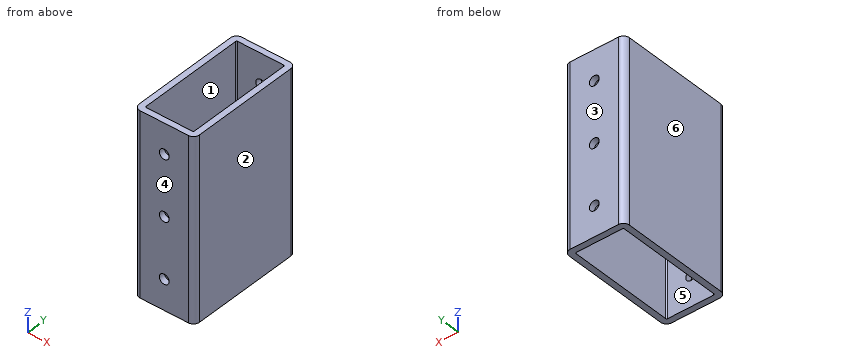
```python
from build123d import *

# Parameters (mm, degrees)
SKETCH1_W                 = 76.2
SKETCH1_H                 = 50.8
BOSS_EXTRUDE1_DEPTH       = 25.4
SKETCH2_W                 = 20.32
SKETCH2_H                 = 45.72
CUT_EXTRUDE1_DEPTH        = 77.2
F_6_CLEARANCE_HOLE1_D     = 4.1402
F_6_CLEARANCE_HOLE1_DEPTH = 50.8
F_6_CLEARANCE_HOLE2_D     = 4.1402
F_6_CLEARANCE_HOLE2_DEPTH = 50.8
FILLET1_R                 = 0.5
FILLET2_R                 = 2.54


with BuildPart() as part:
    # Sketch1 → Boss-Extrude1 (new body)
    with BuildSketch(Plane(origin=(12.7, 0, 0), x_dir=(0, 0, -1), z_dir=(1, 0, 0))):
        Rectangle(SKETCH1_W, SKETCH1_H)
    extrude(amount=-BOSS_EXTRUDE1_DEPTH)

    # Sketch2 → Cut-Extrude1 (cut, through all)
    with BuildSketch(Plane(origin=(0, 0, -38.1), x_dir=(-1, 0, 0), z_dir=(0, 0, -1))):
        Rectangle(SKETCH2_W, SKETCH2_H)
    extrude(amount=-CUT_EXTRUDE1_DEPTH, mode=Mode.SUBTRACT)

    # #6 Clearance Hole1
    with Locations(Plane(origin=(0, -25.4, 0), x_dir=(-1, 0, 0), z_dir=(0, -1, 0))):
        with Locations((0, 711.2), (0, 736.6), (0, 685.8), (0, 660.4), (0, 635), (0, 609.6), (0, 584.2), (0, 558.8), (0, 533.4), (0, 508), (0, 482.6), (0, 457.2), (0, 431.8), (0, 406.4), (0, 381), (0, 355.6), (0, 330.2), (0, 304.8), (0, 279.4), (0, 254), (0, 228.6), (0, 203.2), (0, 177.8), (0, 152.4), (0, 127), (0, 101.6), (0, 76.2), (0, 50.8), (0, 25.4), (0, 0), (0, -25.4), (0, -50.8), (0, -76.2), (0, -101.6), (0, -127), (0, -152.4), (0, -177.8), (0, -203.2), (0, -228.6), (0, -254), (0, -279.4), (0, -304.8), (0, -330.2), (0, -355.6), (0, -381), (0, -406.4), (0, -431.8), (0, -457.2), (0, -482.6), (0, -508), (0, -533.4), (0, -558.8), (0, -584.2), (0, -609.6), (0, -635), (0, -660.4), (0, -685.8), (0, -711.2), (0, -736.6)):
            Hole(F_6_CLEARANCE_HOLE1_D / 2, depth=F_6_CLEARANCE_HOLE1_DEPTH)

    # #6 Clearance Hole2
    with Locations(Plane(origin=(0, 25.4, 0), x_dir=(1, 0, 0), z_dir=(0, 1, 0))):
        with Locations((0, 711.2), (0, 736.6), (0, 685.8), (0, 660.4), (0, 635), (0, 609.6), (0, 584.2), (0, 558.8), (0, 533.4), (0, 508), (0, 482.6), (0, 457.2), (0, 431.8), (0, 406.4), (0, 381), (0, 355.6), (0, 330.2), (0, 304.8), (0, 279.4), (0, 254), (0, 228.6), (0, 203.2), (0, 177.8), (0, 152.4), (0, 127), (0, 101.6), (0, 76.2), (0, 50.8), (0, 25.4), (0, 0), (0, -25.4), (0, -50.8), (0, -76.2), (0, -101.6), (0, -127), (0, -152.4), (0, -177.8), (0, -203.2), (0, -228.6), (0, -254), (0, -279.4), (0, -304.8), (0, -330.2), (0, -355.6), (0, -381), (0, -406.4), (0, -431.8), (0, -457.2), (0, -482.6), (0, -508), (0, -533.4), (0, -558.8), (0, -584.2), (0, -609.6), (0, -635), (0, -660.4), (0, -685.8), (0, -711.2), (0, -736.6)):
            Hole(F_6_CLEARANCE_HOLE2_D / 2, depth=F_6_CLEARANCE_HOLE2_DEPTH)

    # Fillet1
    fillet1_edges = [part.edges().sort_by_distance(p)[0] for p in [
        (-10.16, -22.86, 0),
        (10.16, -22.86, 0),
        (10.16, 22.86, 0),
        (-10.16, 22.86, 0),
    ]]
    fillet(fillet1_edges, radius=FILLET1_R)

    # Fillet2
    fillet2_edges = [part.edges().sort_by_distance(p)[0] for p in [
        (-12.7, 25.4, 0),
        (-12.7, -25.4, 0),
        (12.7, 25.4, 0),
        (12.7, -25.4, 0),
    ]]
    fillet(fillet2_edges, radius=FILLET2_R)


solid = part.part
```
CAD build for the part. Positions are in the model's coordinates, mm. Face numbers are marked on the shaded views. A direction names the side the tool comes from. Give positions to 0.01 mm unless a question says otherwise; leave off trailing zeros. Write each loop counter-clockwise with the first axis right and the second up, starting at its lowest first coordinate (ties: lowest second). Pieces come first, ordered by that corner, then holes. Notation, with made-up numbers: M -34.75,43 L 7.25,43 A15 cw 7.25,65 Z; hole C 15.5,-35 d3. An arc over 180 degrees is marked long. Return JSON: item names as keys, results as strings. Group by question number.
(1) Band-saw the part on C-C (x = -8.25). Give the cut face in (y, z), and give its area (3 significant figures).
(2) Flat gauge pin, fed straight in: pin 1 Ø5 at (x, y) = (-7, 13) entering from +Z. Where does the tip first touch, or does it go through?
(3) Band-saw the part on D-D (x = 0). State how many separate pieces and enclosed holes the cut face has, and give its area (3 significant figures).
(4) Band-saw the part on B-B (y = 7). Give the cut face in (x, z).
(5) Drill centre lines: L1, parallel to Z at x = 0, y = -24.2; L2, parallel to Y at x = 7.25, z = -8.5; L3, parallel to X at y = 12, z = 26.5. Where is each one in solid material? Low to high. Write a range as [from, to].
(6) Mould opens along Y. For the marked faces 3, 4, 5 and 6 say: pulls with the +Y half, pulls with the -Y half, needs draft (parallel to the pull), parting line crosses it, or undercut.
(7) Band-saw the part on A-A (z = 25.4). Give the cut face in (x, y).
(8) 3-axis set-ups, long thin cutter, end or side, ignore diameter. For the marked faces 1 and 2: which of +Z, -Z, +X, -X, +Y, -Y reach the whole face in a straight line?
Entries:
{
 "1": {"outline": "M -25.4,-38.1 L -22.86,-38.1 L -22.86,38.1 L -25.4,38.1 Z; M 22.86,-38.1 L 25.4,-38.1 L 25.4,38.1 L 22.86,38.1 Z", "area": "387 mm^2"},
 "2": {"pin 1": "passes through"},
 "3": {"separate pieces": "8", "enclosed holes": "0", "area": "324 mm^2"},
 "4": {"outline": "M -12.7,-38.1 L -10.16,-38.1 L -10.16,38.1 L -12.7,38.1 Z; M 10.16,-38.1 L 12.7,-38.1 L 12.7,38.1 L 10.16,38.1 Z"},
 "5": {"L1": "z = [-38.1, -27.47], [-23.33, -2.07], [2.07, 23.33], [27.47, 38.1]", "L2": "y = [-25.4, -22.86], [22.86, 25.4]", "L3": "x = [-12.7, -10.16], [10.16, 12.7]"},
 "6": {"face 3": "pulls with the +Y half", "face 4": "pulls with the -Y half", "face 5": "undercut", "face 6": "needs draft"},
 "7": {"outline": "M -12.7,-22.86 A2.54 ccw -10.16,-25.4 L -2.07,-25.4 L -2.07,-22.86 L -9.66,-22.86 A0.5 cw -10.16,-22.36 L -10.16,22.36 A0.5 cw -9.66,22.86 L -2.07,22.86 L -2.07,25.4 L -10.16,25.4 A2.54 ccw -12.7,22.86 Z; M 2.07,-25.4 L 10.16,-25.4 A2.54 ccw 12.7,-22.86 L 12.7,22.86 A2.54 ccw 10.16,25.4 L 2.07,25.4 L 2.07,22.86 L 9.66,22.86 A0.5 cw 10.16,22.36 L 10.16,-22.36 A0.5 cw 9.66,-22.86 L 2.07,-22.86 Z"},
 "8": {"face 1": "+Z, -Z", "face 2": "+Z, -Z, +X, +Y, -Y"}
}
